from build123d import *

# Parameters (mm, degrees)
SKETCH1_W           = 500
SKETCH1_H           = 290
SKETCH1_R           = 2.5
SKETCH1_R_2         = 17.5
SKETCH1_R_3         = 12.5
SKETCH1_R_4         = 2
BOSS_EXTRUDE1_DEPTH = 10


with BuildPart() as part:
    # Sketch1 → Boss-Extrude1 (new body)
    with BuildSketch(Plane(origin=(0, 0, 0), x_dir=(1, 0, 0), z_dir=(0, 1, 0))):
        Rectangle(SKETCH1_W, SKETCH1_H)
        with Locations((-240, 0)):
            Circle(SKETCH1_R, mode=Mode.SUBTRACT)
        with Locations((-90, 0)):
            Circle(SKETCH1_R, mode=Mode.SUBTRACT)
        with Locations((-170, -135)):
            Circle(SKETCH1_R, mode=Mode.SUBTRACT)
        with Locations((-170, 135)):
            Circle(SKETCH1_R, mode=Mode.SUBTRACT)
        with Locations((170, 135)):
            Circle(SKETCH1_R, mode=Mode.SUBTRACT)
        with Locations((240, 0)):
            Circle(SKETCH1_R, mode=Mode.SUBTRACT)
        with Locations((170, -135)):
            Circle(SKETCH1_R, mode=Mode.SUBTRACT)
        with Locations((0, 135)):
            Circle(SKETCH1_R, mode=Mode.SUBTRACT)
        with Locations((0, -135)):
            Circle(SKETCH1_R, mode=Mode.SUBTRACT)
        with Locations((100, 0)):
            Circle(SKETCH1_R_2, mode=Mode.SUBTRACT)
        with Locations((-140, 0)):
            Circle(SKETCH1_R_3, mode=Mode.SUBTRACT)
        with Locations((-125.857864376, 14.142135624)):
            Circle(SKETCH1_R, mode=Mode.SUBTRACT)
        with Locations((-125.857864376, -14.142135624)):
            Circle(SKETCH1_R, mode=Mode.SUBTRACT)
        with Locations((-154.142135624, -14.142135624)):
            Circle(SKETCH1_R, mode=Mode.SUBTRACT)
        with Locations((-154.142135624, 14.142135624)):
            Circle(SKETCH1_R, mode=Mode.SUBTRACT)
        with Locations((170, 0)):
            Circle(SKETCH1_R, mode=Mode.SUBTRACT)
        with Locations((131.819805153, 31.819805153)):
            Circle(SKETCH1_R_4, mode=Mode.SUBTRACT)
        with Locations((100, -70)):
            Circle(SKETCH1_R, mode=Mode.SUBTRACT)
        with Locations((30, 0)):
            Circle(SKETCH1_R, mode=Mode.SUBTRACT)
        with Locations((100, 70)):
            Circle(SKETCH1_R, mode=Mode.SUBTRACT)
        with Locations((131.819805153, -31.819805153)):
            Circle(SKETCH1_R_4, mode=Mode.SUBTRACT)
        with Locations((68.180194847, -31.819805153)):
            Circle(SKETCH1_R_4, mode=Mode.SUBTRACT)
        with Locations((68.180194847, 31.819805153)):
            Circle(SKETCH1_R_4, mode=Mode.SUBTRACT)
    extrude(amount=BOSS_EXTRUDE1_DEPTH)


solid = part.part
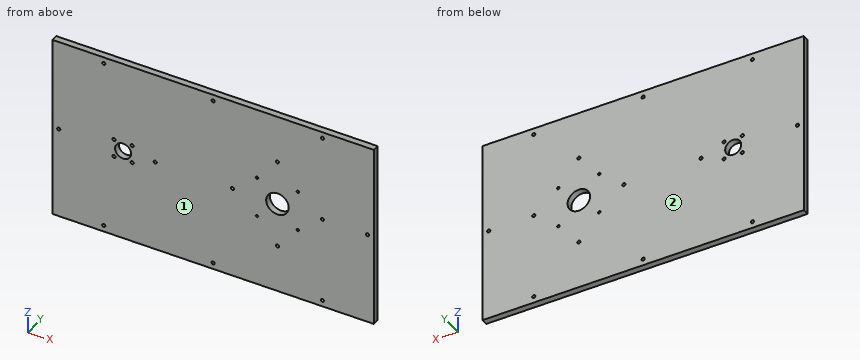
Design review of the part built by this model. Coordinates are the model's own, in mm. Face numbers are marked on the shaded views. Give positions to 0.01 mm unless a question says otherwise; leave off trailing zeros. One line per question, with ' | ' between items. Start each with the question number.
1. Insertion check: P1, Ø8, axis at x = 100, z = -70, coming from the +Y side. The pin has a flat end and moves straight along its axis. Give the tip position at first contact, or say it passes through.
2. The part is to be moulded in two halves that separate along Y. For the marked faces 1 and 2, say which applies: released by +Y, released by -Y, zero draft, split by the parting line, or undercut.
3. To check wall thickness, follow L1, parallel to X at y = 7, z = -135; L2, parallel to Z at x = 100, y = 7; L3, parallel to Z at x = 170, y = 4. State the ranges of each line that lie inside material, in increasing order.
Worked out:
1) P1: stops at y = 10
2) face 1: released by -Y | face 2: released by +Y
3) L1: x = -250 to -172.5, -167.5 to -2.5, 2.5 to 167.5, 172.5 to 250 | L2: z = -145 to -72.5, -67.5 to -17.5, 17.5 to 67.5, 72.5 to 145 | L3: z = -145 to -137.5, -132.5 to -2.5, 2.5 to 132.5, 137.5 to 145
